Check sheet for the drawn part. Datum: minimum x, y, z corner. Units: mm. A direction names the side the tool comes from. Give positions to 0.01 mm unless a question says otherwise; leave off trailing zeros. Write each loop counter-clockwise with the first axis right and the second up, starting at its lowest first coordinate (ties: lowest second). Pieces come first, ordered by that corner, then holes. Notation, with made-up numbers: (-7.75, -15) - (39.25, -15) arc R24 cw to (39.25, -1) - close; hole circle Ø10 at (29, -24). An arc over 180 degrees is marked (long way). Use a Markdown table: item, result.
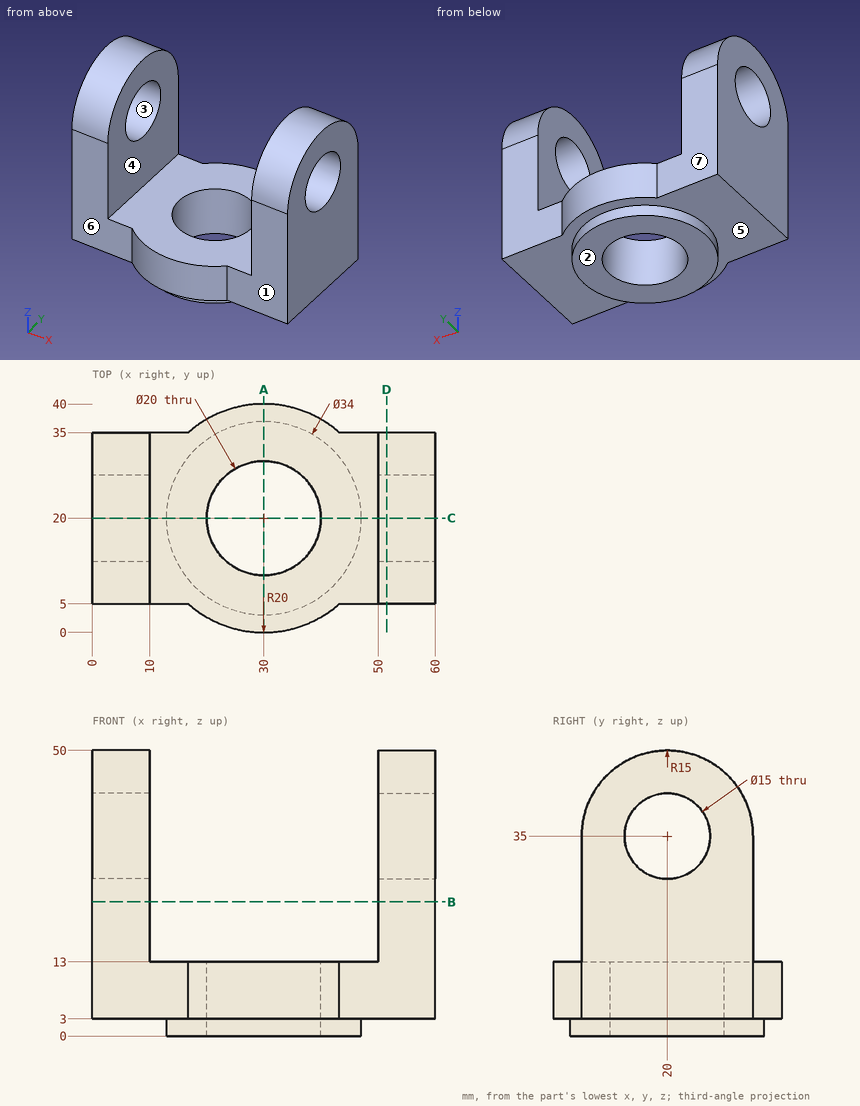
1) Depth check by flat-ended pin: P1, Ø20, axis at x = 33.5, y = 20, coming from the +Z side; P2, Ø24, axis at y = 14.5, z = 28.5, coming from the -X side; P3, Ø5, axis at x = 50, y = 20, coming from the -Z side; P4, Ø2, axis at y = 26, z = 35, coming from the -X side. Enter the tip coordinate at first touch or a pass-through.
Working result:
| item | result |
|---|---|
| P1 | stops at z = 13 |
| P2 | stops at x = 0 |
| P3 | stops at z = 3 |
| P4 | passes through |
2) Material ranges on L1, parallel to X at y = 29, z = 28.5; L2, parallel to Z at x = 6.5, y = 20; L3, parallel to Z at x = 36.5, y = 7.5, recorded low to high. Write a range as from..to.
Working result:
| item | result |
|---|---|
| L1 | x = 0..10, 50..60 |
| L2 | z = 3..27.5, 42.5..50 |
| L3 | z = 0..13 |
3) Set-up check for the marked faces 4, 5, 6 and 7: record each of +Z, -Z, +X, -X, +Y, -Y from which the full face is reachable in a straight line by a thin tool's end or side.
Working result:
| item | result |
|---|---|
| face 4 | +Z, +Y, -Y |
| face 5 | -Z |
| face 6 | +Z, -Z, -X, -Y |
| face 7 | +Z, -Z, -X, +Y |
4) Section check B-B on z = 23.5. Record the boundary of the cut face in (x, y), then the cut area to 3 significant figures.
Working result:
| item | result |
|---|---|
| outline | (0, 5) - (10, 5) - (10, 35) - (0, 35) - close; (50, 5) - (60, 5) - (60, 35) - (50, 35) - close |
| area | 600 mm² |
5) Section check D-D on x = 51.5. Record the boundary of the cut face in (y, z), then the cut area to 3 significant figures.
Working result:
| item | result |
|---|---|
| outline | (5, 3) - (35, 3) - (35, 35) arc R15 ccw to (5, 35) - close; hole circle Ø15 at (20, 35) |
| area | 1,140 mm² |
6) Section check A-A on x = 30. Record the boundary of the cut face in (y, z).
Working result:
| item | result |
|---|---|
| outline | (0, 3) - (3, 3) - (3, 0) - (10, 0) - (10, 13) - (0, 13) - close; (30, 0) - (37, 0) - (37, 3) - (40, 3) - (40, 13) - (30, 13) - close |
7) Mould release check, pull along Y, two halves, no side actions. Record for the marked faces 1, 2 and 3: pulls with the +Y half, pulls with the -Y half, needs draft (parallel to the pull), parting line crosses it, or undercut.
Working result:
| item | result |
|---|---|
| face 1 | pulls with the -Y half |
| face 2 | needs draft |
| face 3 | undercut |
8) Section check C-C on y = 20. Record the boundary of the cut face in (x, z), then the cut area to 3 significant figures.
Working result:
| item | result |
|---|---|
| outline | (0, 3) - (13, 3) - (13, 0) - (20, 0) - (20, 13) - (10, 13) - (10, 27.5) - (0, 27.5) - close; (0, 42.5) - (10, 42.5) - (10, 50) - (0, 50) - close; (40, 0) - (47, 0) - (47, 3) - (60, 3) - (60, 27.5) - (50, 27.5) - (50, 13) - (40, 13) - close; (50, 42.5) - (60, 42.5) - (60, 50) - (50, 50) - close |
| area | 882 mm² |
